The model under review builds one solid part; all positions refer to its coordinate system, in mm. Coordinates: 2 decimals unless noted, no trailing zeros. Order: outer loops, then holes, each group sorted by start corner. A loop starts at its lowest first (then second) coordinate and runs counter-clockwise, first axis right, second up. Notation, with made-up numbers: M 35,44.25 L 49,44.25 A12 cw 49,57.25 Z; hole C 36.5,59 d8. An arc over 180 degrees is marked long. One line per item, written item: value.
```python
from build123d import *

# Parameters (mm, degrees)
SKETCH1_R           = 6.5
SKETCH1_R_2         = 1.5
BOSS_EXTRUDE1_DEPTH = 1.5875
FILLET2_R           = 13
CHAMFER1_SIZE       = 30


with BuildPart() as part:
    # Sketch1 → Boss-Extrude1 (new body)
    with BuildSketch(Plane.XY):
        Polygon((0, 0), (0, 50), (0, 79.5), (97.5, 79.5), (97.5, 39.5), (35, 39.5), (35, 0), (35, -26), (0, -26), align=None)
        with Locations((17.5, -13)):
            Circle(SKETCH1_R, mode=Mode.SUBTRACT)
        with Locations((77.5, 59.5)):
            Circle(SKETCH1_R, mode=Mode.SUBTRACT)
        with Locations((17.5, 45)):
            Circle(SKETCH1_R_2, mode=Mode.SUBTRACT)
        with Locations((17.5, 25)):
            Circle(SKETCH1_R_2, mode=Mode.SUBTRACT)
        with Locations((17.5, 5)):
            Circle(SKETCH1_R_2, mode=Mode.SUBTRACT)
    extrude(amount=BOSS_EXTRUDE1_DEPTH)

    # Fillet2
    fillet2_edges = [part.edges().sort_by_distance(p)[0] for p in [
        (97.5, 79.5, 0.79375),
        (97.5, 39.5, 0.79375),
        (35, -26, 0.79375),
        (0, -26, 0.79375),
    ]]
    fillet(fillet2_edges, radius=FILLET2_R)

    # Chamfer1
    chamfer1_edges = [part.edges().sort_by_distance(p)[0] for p in [
        (0, 79.5, 0.79375),
        (35, 39.5, 0.79375),
    ]]
    chamfer(chamfer1_edges, length=CHAMFER1_SIZE)


solid = part.part
```
(1) Mouldability with a two-part tool opening along X and no side actions: class faces 1 (the cylindrical face through (17.175, 43.536, 0.783)), 2 (the flat face through (39, 39, 1.588)), 3 (the flat face through (15.2, 64.7, 0.8)) as +X half, -X half, draft (parallel to the pull), parting line (faces both ways), or undercut.
Geometry results:
face 1: undercut
face 2: draft
face 3: -X half
(2) We need section A-A, the plane x = 77.5. State the section outline as (y, z) points.
Geometry results:
outline: M 39.5,0 L 53,0 L 53,1.59 L 39.5,1.59 Z; M 66,0 L 79.5,0 L 79.5,1.59 L 66,1.59 Z
(3) Insertion check: pin 1 Ø0.5 at (x, z) = (74.5, 1) entering from -Y. The pin has a flat end and moves straight along its axis. Give the tip position at first contact, or say it passes through.
Geometry results:
pin 1: stops at y = 39.5
(4) For L1, parallel to Y at x = 17.5, z = 0.85; L2, parallel to X at y = -14.5, z = 0.9; L3, parallel to Y at x = 65, z = 0.1, list the stretches that pass through material, from the lowest coordinate up.
Geometry results:
L1: y = -26 to -19.5, -6.5 to 3.5, 6.5 to 23.5, 26.5 to 43.5, 46.5 to 67
L2: x = 0.09 to 11.18, 23.82 to 34.91
L3: y = 39.5 to 79.5
(5) We need section B-B, the plane y = 25. State the section outline as (x, z) points, plus the area to 3 significant figures.
Geometry results:
outline: M 0,0 L 16,0 L 16,1.59 L 0,1.59 Z; M 19,0 L 50.5,0 L 50.5,1.59 L 19,1.59 Z
area: 75.4 mm2
(6) We need section C-C, the plane x = 17.5. State the section outline as (y, z) points, plus the area to 3 significant figures.
Geometry results:
outline: M -26,0 L -19.5,0 L -19.5,1.59 L -26,1.59 Z; M -6.5,0 L 3.5,0 L 3.5,1.59 L -6.5,1.59 Z; M 6.5,0 L 23.5,0 L 23.5,1.59 L 6.5,1.59 Z; M 26.5,0 L 43.5,0 L 43.5,1.59 L 26.5,1.59 Z; M 46.5,0 L 67,0 L 67,1.59 L 46.5,1.59 Z
area: 113 mm2
(7) We need section D-D, the plane z = 1.2. State the section outline as (x, y) points.
Geometry results:
outline: M 0,-13 A13 ccw 13,-26 L 22,-26 A13 ccw 35,-13 L 35,9.5 L 65,39.5 L 84.5,39.5 A13 ccw 97.5,52.5 L 97.5,66.5 A13 ccw 84.5,79.5 L 30,79.5 L 0,49.5 Z; hole C 17.5,-13 d13; hole C 17.5,5 d3; hole C 17.5,25 d3; hole C 17.5,45 d3; hole C 77.5,59.5 d13
